```python
from build123d import *

# Parameters (mm, degrees)
F0_W     = 152.4
F0_H     = 152.4
F1_DEPTH = 152.4
F2_R     = 25.4
F3_DEPTH = 152.401
F4_R     = 25.4
F5_DEPTH = 152.401
F6_R     = 25.4
F7_DEPTH = 152.401


with BuildPart() as f1:
    # F0 (on Top) → F1 (new body)
    with BuildSketch(Plane.XY):
        Rectangle(F0_W, F0_H)
    extrude(amount=F1_DEPTH)

    # F2 (on face) → F3 (cut, through all)
    with BuildSketch(Plane.YZ.offset(76.2)):
        with Locations((0, 76.2)):
            Circle(F2_R)
    extrude(amount=-F3_DEPTH, mode=Mode.SUBTRACT)

    # F4 (on face) → F5 (cut, through all)
    with BuildSketch(Plane(origin=(0, 76.2, 0), x_dir=(-1, 0, 0), z_dir=(0, 1, 0))):
        with Locations((0, 76.2)):
            Circle(F4_R)
    extrude(amount=-F5_DEPTH, mode=Mode.SUBTRACT)

    # F6 (on face) → F7 (cut, through all)
    with BuildSketch(Plane.XY.offset(152.4)):
        Circle(F6_R)
    extrude(amount=-F7_DEPTH, mode=Mode.SUBTRACT)


solid = f1.part
```
Geometry check sheet. Reference: the model listing, model coordinates, mm. Round coordinates to 2 decimals unless told otherwise and drop trailing zeros. Write each loop counter-clockwise with the first axis right and the second up, starting at its lowest first coordinate (ties: lowest second). Pieces come first, ordered by that corner, then holes. Notation, with made-up numbers: (-29, 64) - (24, 64) arc R22 cw to (24, 88) - close; hole circle Ø8 at (-31.75, 14.25). An arc over 180 degrees is marked (long way). Write each question's results on one line, items separated by ' | '.
(1) Sectioned sample at C-C, the plane y = 38. Enter the section's corners in (x, z), plus the area to 3 significant figures.
Computed:
outline: (-76.2, 0) - (76.2, 0) - (76.2, 152.4) - (-76.2, 152.4) - close; hole circle Ø50.8 at (0, 76.2) | area: 21,200 mm^2
(2) Sectioned sample at A-A, the plane z = 76.2. Enter the section's corners in (x, y), plus the area to 3 significant figures.
Computed:
outline: (-76.2, -76.2) - (-25.4, -76.2) - (-25.4, -25.4) - (-76.2, -25.4) - close; (-76.2, 25.4) - (-25.4, 25.4) - (-25.4, 76.2) - (-76.2, 76.2) - close; (25.4, -76.2) - (76.2, -76.2) - (76.2, -25.4) - (25.4, -25.4) - close; (25.4, 25.4) - (76.2, 25.4) - (76.2, 76.2) - (25.4, 76.2) - close | area: 10,300 mm^2
(3) Thickness scan on probe 1 along Z at (x, y) = (0, -36.5); probe 2 along Y at (x, z) = (42, 76); probe 3 along X at (y, z) = (-42, 61). Record the ranges inside material, lowest first. Write a range as from..to.
Computed:
probe 1: z = 0..50.8, 101.6..152.4 | probe 2: y = -76.2..-25.4, 25.4..76.2 | probe 3: x = -76.2..-20.35, 20.35..76.2
(4) Sectioned sample at B-B, the plane x = 0. Enter the section's corners in (y, z), plus the area to 3 significant figures.
Computed:
outline: (-76.2, 0) - (-25.4, 0) - (-25.4, 50.8) - (-76.2, 50.8) - close; (-76.2, 101.6) - (-25.4, 101.6) - (-25.4, 152.4) - (-76.2, 152.4) - close; (25.4, 0) - (76.2, 0) - (76.2, 50.8) - (25.4, 50.8) - close; (25.4, 101.6) - (76.2, 101.6) - (76.2, 152.4) - (25.4, 152.4) - close | area: 10,300 mm^2
(5) Sectioned sample at D-D, the plane z = 138. Enter the section's corners in (x, y).
Computed:
outline: (-76.2, -76.2) - (76.2, -76.2) - (76.2, 76.2) - (-76.2, 76.2) - close; hole circle Ø50.8 at (0, 0)
(6) Draft check along Z on faces 1 (the face through (-1, 35, 152.4)), 2 (the face through (-76.2, -18, 58)), 3 (the face through (-1, 35, 0)), 4 (the face through (-46.673, -25.375, 77.317)). Enter one of: pulls with the +Z half, pulls with the -Z half, needs draft (parallel to the pull), parting line crosses it, or undercut.
Computed:
face 1: pulls with the +Z half | face 2: needs draft | face 3: pulls with the -Z half | face 4: undercut
